Source: CAD feature listing. Evaluate the final solid. Frame: model axes, mm. A direction names the side the tool comes from. Give positions to 0.01 mm unless a question says otherwise; leave off trailing zeros. Loops run counter-clockwise (first coordinate to the right, second up) from the corner with the lowest first, then second, coordinate; pieces in that order, holes last. Notation, with made-up numbers: (68, 71.5) -> (115, 71.5) arc R15 ccw to (115, 89.5) -> close; hole circle Ø11 at (80, 59). An arc over 180 degrees is marked (long way). Put each result on its own line as item: value.
```python
from build123d import *

# Parameters (mm, degrees)
F0_W     = 120
F0_H     = 10
F0_R     = 1.5
F1_DEPTH = 2
F2_W     = 6
F2_H     = 30
F3_DEPTH = 4


with BuildPart() as f1:
    # F0 (on Top) → F1 (new body, symmetric)
    with BuildSketch(Plane.XY):
        with Locations((60, 5)):
            Rectangle(F0_W, F0_H)
        with Locations((16, 5)):
            Circle(F0_R, mode=Mode.SUBTRACT)
        with Locations((104, 5)):
            Circle(F0_R, mode=Mode.SUBTRACT)
    extrude(amount=F1_DEPTH, both=True)

    # F2 (on face) → F3 (join)
    with BuildSketch(Plane(origin=(0, 10, 0), x_dir=(-1, 0, 0), z_dir=(0, 1, 0))):
        with BuildLine():
            Line((-63, 32), (-57, 32))
            Line((-57, 32), (-37, 32))
            ThreePointArc((-37, 32), (-33.4644660941, 33.4644660941), (-32, 37))
            Line((-32, 37), (-32, 40))
            ThreePointArc((-32, 40), (-33.4644660941, 43.5355339059), (-37, 45))
            Line((-37, 45), (-83, 45))
            ThreePointArc((-83, 45), (-86.5355339059, 43.5355339059), (-88, 40))
            Line((-88, 40), (-88, 37))
            ThreePointArc((-88, 37), (-86.5355339059, 33.4644660941), (-83, 32))
            Line((-83, 32), (-63, 32))
        make_face()
        with BuildLine():
            ThreePointArc((-84, 40), (-83.7071067812, 40.7071067812), (-83, 41))
            Line((-83, 41), (-37, 41))
            ThreePointArc((-37, 41), (-36.2928932188, 40.7071067812), (-36, 40))
            Line((-36, 40), (-36, 37))
            ThreePointArc((-36, 37), (-36.2928932188, 36.2928932188), (-37, 36))
            Line((-37, 36), (-83, 36))
            ThreePointArc((-83, 36), (-83.7071067812, 36.2928932188), (-84, 37))
            Line((-84, 37), (-84, 40))
        make_face(mode=Mode.SUBTRACT)
        with Locations((-60, 17)):
            Rectangle(F2_W, F2_H)
    extrude(amount=-F3_DEPTH)


solid = f1.part
```
(1) Section B-B on x = 16. Return loops of the section in (y, z).
Calculated:
outline: (0, -2) -> (3.5, -2) -> (3.5, 2) -> (0, 2) -> close; (6.5, -2) -> (10, -2) -> (10, 2) -> (6.5, 2) -> close
(2) Section C-C on y = 8.75. Return loops of the section in (x, z), then the cut area to 3 significant figures.
Calculated:
outline: (0, -2) -> (120, -2) -> (120, 2) -> (63, 2) -> (63, 32) -> (83, 32) arc R5 ccw to (88, 37) -> (88, 40) arc R5 ccw to (83, 45) -> (37, 45) arc R5 ccw to (32, 40) -> (32, 37) arc R5 ccw to (37, 32) -> (57, 32) -> (57, 2) -> (0, 2) -> close; hole (36, 37) arc R1 ccw to (37, 36) -> (83, 36) arc R1 ccw to (84, 37) -> (84, 40) arc R1 ccw to (83, 41) -> (37, 41) arc R1 ccw to (36, 40) -> close
area: 1,130 mm²
(3) Section A-A on x = 81. Return loops of the section in (y, z), then the cut area to 3 significant figures.
Calculated:
outline: (0, -2) -> (10, -2) -> (10, 2) -> (0, 2) -> close; (6, 32) -> (10, 32) -> (10, 36) -> (6, 36) -> close; (6, 41) -> (10, 41) -> (10, 45) -> (6, 45) -> close
area: 72.0 mm²
(4) Section D-D on z = 8. Return loops of the section in (x, y).
Calculated:
outline: (57, 6) -> (63, 6) -> (63, 10) -> (57, 10) -> close
(5) First-contact query: P1, Ø8, axis at x = 59.5, z = 8.5, coming from the -Y side; P2, Ø1.5, axis at y = 7.5, z = 39, coming from the +X side; P3, Ø3, axis at y = 7.5, z = 14.5, coming from the +X side; P4, Ø3.5, axis at x = 104, y = 5, coming from the -Z side. Flat tips, straight axial feed; report the tip coordinate or a pass-through.
Calculated:
P1: stops at y = 6
P2: stops at x = 88
P3: stops at x = 63
P4: stops at z = -2
(6) Reachability of faces 4 (the flat face through (47, 8, 32)), 5 (the flat face through (88, 8, 39)), 6 (the flat face through (36, 8, 39)), 7 (the flat face through (32, 8, 38)), 8 (the flat face through (63, 8, 17)) from +Z, -Z, +X, -X, +Y, -Y: full face, straight path, thin tool, end or side. Return the list, or none.
Calculated:
face 4: -X, +Y, -Y
face 5: +Z, +X, +Y, -Y
face 6: +Y, -Y
face 7: +Z, -X, +Y, -Y
face 8: +X, +Y, -Y
(7) Line query: probe 1 along Z at (x, y) = (42, 9); probe 2 along Z at (x, y) = (84.5, 4); probe 3 along Z at (x, y) = (84.5, 7.5). Output: solid intervals per line, ascending. Write a range as from..to.
Calculated:
probe 1: z = -2..2, 32..36, 41..45
probe 2: z = -2..2
probe 3: z = -2..2, 32.23..44.77
(8) Draft query along Y for faces 1 (the cylindrical face through (14.5, 5.07, -0.03)), 2 (the flat face through (60, 10, 20)), 3 (the flat face through (73, 8, 32)). Return one class per face: released by +Y, released by -Y, zero draft, split by the parting line, or undercut.
Calculated:
face 1: undercut
face 2: released by +Y
face 3: zero draft
